from build123d import *

# Parameters (mm, degrees)
SKETCH1_W           = 46.2
SKETCH1_H           = 13
BOSS_EXTRUDE1_DEPTH = 1.5
SKETCH3_R           = 1
CUT_EXTRUDE1_DEPTH  = 25.183878928
SKETCH4_W           = 23.7
SKETCH4_H           = 8.5
CUT_EXTRUDE2_DEPTH  = 25.183878928
FILLET1_R           = 3


with BuildPart() as part:
    # Sketch1 → Boss-Extrude1 (new, symmetric)
    with BuildSketch(Plane(origin=(0, 0, 0), x_dir=(1, 0, 0), z_dir=(0, 1, 0))):
        Rectangle(SKETCH1_W, SKETCH1_H)
    extrude(amount=BOSS_EXTRUDE1_DEPTH, both=True)

    # Sketch3 → Cut-Extrude1 (cut, through all)
    with BuildSketch(Plane(origin=(0, 1.5, 0), x_dir=(1, 0, 0), z_dir=(0, 1, 0))):
        with Locations(Location((-21.1, 4.5, 0), (0, 0, 270))):
            Circle(SKETCH3_R)
        with Locations(Location((-6.6, 4.5, 0), (0, 0, 270))):
            Circle(SKETCH3_R)
        with Locations(Location((21.1, 4.5, 0), (0, 0, 270))):
            Circle(SKETCH3_R)
    extrude(amount=-CUT_EXTRUDE1_DEPTH, mode=Mode.SUBTRACT)

    # Sketch4 → Cut-Extrude2 (cut, through all)
    with BuildSketch(Plane(origin=(0, 1.5, 0), x_dir=(1, 0, 0), z_dir=(0, 1, 0))):
        with Locations((7.25, 2.25)):
            Rectangle(SKETCH4_W, SKETCH4_H)
    extrude(amount=-CUT_EXTRUDE2_DEPTH, mode=Mode.SUBTRACT)

    # Fillet1
    fillet1_edges = [part.edges().sort_by_distance(p)[0] for p in [
        (-4.6, 0, 2),
        (19.1, 0, 2),
    ]]
    fillet(fillet1_edges, radius=FILLET1_R)


solid = part.part
Could you check a few things on this model? Use its own coordinates, in mm. A direction names the side the tool comes from. Give positions to 0.01 mm unless a question says otherwise; leave off trailing zeros. Order: outer loops, then holes, each group sorted by start corner. A loop starts at its lowest first (then second) coordinate and runs counter-clockwise, first axis right, second up. Notation, with made-up numbers: (18.25, -39) -> (32.25, -39) arc R35 ccw to (32.25, -5) -> close; hole circle Ø8 at (79, -13). An arc over 180 degrees is marked (long way). Return JSON: item names as keys, results as strings.
1. Imagine slicing it at C-C on y = -0.15. List the corners of the cut face in (x, z) for me.
Answer list:
{"outline": "(-23.1, -6.5) -> (-4.6, -6.5) -> (-4.6, -1) arc R3 cw to (-1.6, 2) -> (16.1, 2) arc R3 cw to (19.1, -1) -> (19.1, -6.5) -> (23.1, -6.5) -> (23.1, 6.5) -> (-23.1, 6.5) -> close; hole circle Ø2 at (-21.1, -4.5); hole circle Ø2 at (-6.6, -4.5); hole circle Ø2 at (21.1, -4.5)"}
2. Imagine slicing it at D-D on z = -4. List the corners of the cut face in (x, y) for me, then the cut area to 3 significant figures.
Answer list:
{"outline": "(-23.1, -1.5) -> (-21.97, -1.5) -> (-21.97, 1.5) -> (-23.1, 1.5) -> close; (-20.23, -1.5) -> (-7.47, -1.5) -> (-7.47, 1.5) -> (-20.23, 1.5) -> close; (-5.73, -1.5) -> (-4.6, -1.5) -> (-4.6, 1.5) -> (-5.73, 1.5) -> close; (19.1, -1.5) -> (20.23, -1.5) -> (20.23, 1.5) -> (19.1, 1.5) -> close; (21.97, -1.5) -> (23.1, -1.5) -> (23.1, 1.5) -> (21.97, 1.5) -> close", "area": "51.9 mm2"}
3. For pin 1 Ø0.9 at (x, y) = (5, -0.5) entering from -Z, with a flat end and sliding along its axis, tell me the tip position at first contact or that it passes through.
Answer list:
{"pin 1": "stops at z = 2"}
4. Imagine slicing it at B-B on z = -1.5. List the corners of the cut face in (x, y) for me, then the cut area to 3 significant figures.
Answer list:
{"outline": "(-23.1, -1.5) -> (-4.6, -1.5) -> (-4.6, 1.5) -> (-23.1, 1.5) -> close; (19.1, -1.5) -> (23.1, -1.5) -> (23.1, 1.5) -> (19.1, 1.5) -> close", "area": "67.5 mm2"}
5. Imagine slicing it at A-A on x = 21.1. List the corners of the cut face in (y, z) for me, then the cut area to 3 significant figures.
Answer list:
{"outline": "(-1.5, -6.5) -> (1.5, -6.5) -> (1.5, -5.5) -> (-1.5, -5.5) -> close; (-1.5, -3.5) -> (1.5, -3.5) -> (1.5, 6.5) -> (-1.5, 6.5) -> close", "area": "33.0 mm2"}
6. Thinking about a two-plate mould opening in Z: for faces 1 (the flat face through (7, 0, 2)), 2 (the cylindrical face through (-20.11, 0.02, -4.63)), 3 (the flat face through (-5, -1.5, 1)), which applies, pulls with the +Z half, pulls with the -Z half, needs draft (parallel to the pull), parting line crosses it, or undercut?
Answer list:
{"face 1": "pulls with the -Z half", "face 2": "undercut", "face 3": "needs draft"}
7. On a 3-axis mill with a long thin cutter (end or side, diameter ignored), from which of +Z, -Z, +X, -X, +Y, -Y can I reach the whole of each face in a straight line? I mean faces 4 (the cylindrical face through (18.2, -0.02, 1.14)), 5 (the cylindrical face through (-7.576, 0.021, -4.717)). Say none if no direction works.
Answer list:
{"face 4": "-Z, +Y, -Y", "face 5": "+Y, -Y"}
8. I need wall thicknesses on line 1 (X direction, y = 0.2, z = -4.5); line 2 (X direction, y = -0.95, z = -2); line 3 (Z direction, x = 4.5, y = 1.4). Which ranges of each line are inside material? Lowest first, please. Write a range as from..to.
Answer list:
{"line 1": "x = -23.1..-22.1, -20.1..-7.6, -5.6..-4.6, 19.1..20.1, 22.1..23.1", "line 2": "x = -23.1..-4.6, 19.1..23.1", "line 3": "z = 2..6.5"}
